Source: CAD feature listing. Evaluate the final solid. Frame: model axes, mm. Face numbers are marked on the shaded views. A direction names the side the tool comes from. Coordinates: 2 decimals unless noted, no trailing zeros. Write each loop counter-clockwise with the first axis right and the second up, starting at its lowest first coordinate (ties: lowest second). Pieces come first, ordered by that corner, then holes. Notation, with made-up numbers: (29.25, 71.5) - (43.25, 71.5) arc R19 ccw to (43.25, 93.5) - close; hole circle Ø3 at (6.5, 60.25). An arc over 180 degrees is marked (long way). One line per item, written item: value.
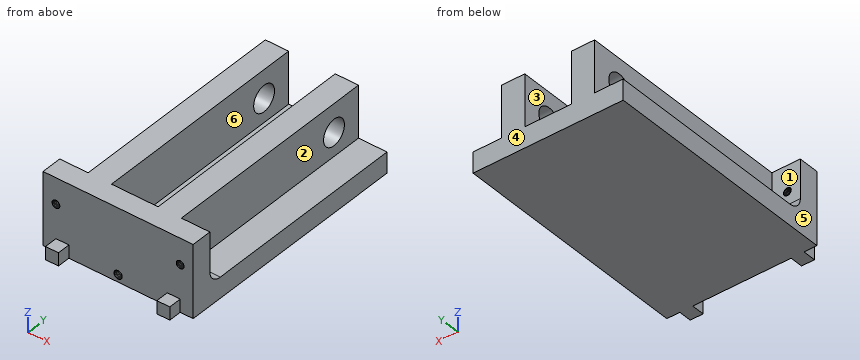
from build123d import *

# Parameters (mm, degrees)
SKETCH1_W           = 57.999998332
SKETCH1_H           = 28.000000864
BOSS_EXTRUDE1_DEPTH = 8
CUT_EXTRUDE2_REACH  = 43.097
CUT_EXTRUDE3_DEPTH  = 42.097445176
CUT_EXTRUDE4_DEPTH  = 42.097445176
SKETCH8_W           = 5.00000082
SKETCH8_H           = 4.999999888
BOSS_EXTRUDE2_DEPTH = 4.999995232
SKETCH9_W           = 5.00000082
SKETCH9_H           = 4.999999888
BOSS_EXTRUDE3_DEPTH = 4.999995232
BOSS_EXTRUDE4_DEPTH = 85
FILLET1_R           = 5
FILLET2_R           = 5
FILLET3_R           = 5
HOLE1_START         = -18
HOLE1_OUTLINE_R     = 5
HOLE1_DEPTH         = 36


# Read off the part's stored shape, not the designer's step: Hole1
with BuildPart() as part:
    # Sketch1 → Boss-Extrude1 (new body)
    with BuildSketch(Plane.XZ):
        with Locations((0, 14.000000432)):
            Rectangle(SKETCH1_W, SKETCH1_H)
    extrude(amount=BOSS_EXTRUDE1_DEPTH)

    # Sketch3 → Cut-Extrude2 (cut, up to next)
    with BuildSketch(Plane.XZ.offset(8), mode=Mode.PRIVATE) as cut_extrude2_sk1:
        Polygon((0, 4.350000061), (-0.277837098, 4.325692076), (-0.547232223, 4.253508057), (-0.79999998, 4.135640804), (-1.028459985, 3.975670785), (-1.225671032, 3.77845997), (-1.385641051, 3.550000023), (-1.503507956, 3.297232091), (-1.575691975, 3.027837025), (-1.59999996, 2.749999985), (-1.575691975, 2.472162945), (-1.503507956, 2.202768112), (-1.385641051, 1.949999947), (-1.225671032, 1.72154), (-1.028459985, 1.524328953), (-0.79999998, 1.36435905), (-0.547232223, 1.246492029), (-0.277837098, 1.17430801), (0, 1.150000026), (0.277837098, 1.17430801), (0.547232223, 1.246492029), (0.79999998, 1.36435905), (1.028459985, 1.524328953), (1.225671032, 1.72154), (1.385641051, 1.949999947), (1.503507956, 2.202768112), (1.575691975, 2.472162945), (1.59999996, 2.749999985), (1.575691975, 3.027837025), (1.503507956, 3.297232091), (1.385641051, 3.550000023), (1.225671032, 3.77845997), (1.028459985, 3.975670785), (0.79999998, 4.135640804), (0.547232223, 4.253508057), (0.277837098, 4.325692076), align=None)
    cut_extrude2_tool1 = extrude(cut_extrude2_sk1.sketch, amount=-CUT_EXTRUDE2_REACH, mode=Mode.PRIVATE) & part.part
    add(cut_extrude2_tool1.solids().sort_by_distance((0, -8, 2.75))[0], mode=Mode.SUBTRACT)

    # Sketch4 → Cut-Extrude3 (cut, through all)
    with BuildSketch(Plane.XZ.offset(8)):
        Polygon((-23.035820574, 16.850929707), (-22.850930691, 17.03581959), (-22.700959817, 17.249999568), (-22.590460256, 17.486970872), (-22.522790357, 17.739530653), (-22.500000894, 17.999999225), (-22.522790357, 18.26046966), (-22.590460256, 18.513029441), (-22.700959817, 18.750000745), (-22.850930691, 18.964180723), (-23.035820574, 19.149070606), (-23.250000551, 19.299039617), (-23.486969993, 19.409539178), (-23.739529774, 19.477209076), (-24.000000209, 19.500000402), (-24.260470644, 19.477209076), (-24.513030425, 19.409539178), (-24.749999866, 19.299039617), (-24.964179844, 19.149070606), (-25.149069726, 18.964180723), (-25.299040601, 18.750000745), (-25.409540161, 18.513029441), (-25.47721006, 18.26046966), (-25.499999523, 17.999999225), (-25.47721006, 17.739530653), (-25.409540161, 17.486970872), (-25.299040601, 17.249999568), (-25.149069726, 17.03581959), (-24.964179844, 16.850929707), (-24.749999866, 16.700960696), (-24.513030425, 16.590459272), (-24.260470644, 16.522789374), (-24.000000209, 16.499999911), (-23.739529774, 16.522789374), (-23.486969993, 16.590459272), (-23.250000551, 16.700960696), align=None)
    extrude(amount=-CUT_EXTRUDE3_DEPTH, mode=Mode.SUBTRACT)

    # Sketch5 → Cut-Extrude4 (cut, through all)
    with BuildSketch(Plane(origin=(0, -8, 0), x_dir=(-1, 0, 0), z_dir=(0, 1, 0))):
        Polygon((-23.486969993, 16.590459272), (-23.250000551, 16.700960696), (-23.035820574, 16.850929707), (-22.850930691, 17.03581959), (-22.700959817, 17.249999568), (-22.590460256, 17.486970872), (-22.522790357, 17.739530653), (-22.500000894, 17.999999225), (-22.522790357, 18.26046966), (-22.590460256, 18.513029441), (-22.700959817, 18.750000745), (-22.850930691, 18.964180723), (-23.035820574, 19.149070606), (-23.250000551, 19.299039617), (-23.486969993, 19.409539178), (-23.739529774, 19.477209076), (-24.000000209, 19.500000402), (-24.260470644, 19.477209076), (-24.513030425, 19.409539178), (-24.749999866, 19.299039617), (-24.964179844, 19.149070606), (-25.149069726, 18.964180723), (-25.299040601, 18.750000745), (-25.409540161, 18.513029441), (-25.47721006, 18.26046966), (-25.499999523, 17.999999225), (-25.47721006, 17.739530653), (-25.409540161, 17.486970872), (-25.299040601, 17.249999568), (-25.149069726, 17.03581959), (-24.964179844, 16.850929707), (-24.749999866, 16.700960696), (-24.513030425, 16.590459272), (-24.260470644, 16.522789374), (-24.000000209, 16.499999911), (-23.739529774, 16.522789374), align=None)
    extrude(amount=CUT_EXTRUDE4_DEPTH, mode=Mode.SUBTRACT)

    # Sketch8 → Boss-Extrude2 (add)
    with BuildSketch(Plane.XZ.offset(8)):
        with Locations((-21.499999799, 2.499999944)):
            Rectangle(SKETCH8_W, SKETCH8_H)
    extrude(amount=BOSS_EXTRUDE2_DEPTH)

    # Sketch9 → Boss-Extrude3 (add)
    with BuildSketch(Plane.XZ.offset(8)):
        with Locations((21.499999799, 2.499999944)):
            Rectangle(SKETCH9_W, SKETCH9_H)
    extrude(amount=BOSS_EXTRUDE3_DEPTH)

    # Sketch10 → Boss-Extrude4 (add)
    with BuildSketch(Plane(origin=(0, 0, 0), x_dir=(1, 0, 0), z_dir=(0, 1, 0))):
        Polygon((9, -8), (-9, -8), (-9, -28.000000864), (-18, -28.000000864), (-18, -8), (-28.999999166, -8), (-28.999999166, 0), (28.999999166, 0), (28.999999166, -8), (18, -8), (18, -28.000000864), (9, -28.000000864), align=None)
    extrude(amount=BOSS_EXTRUDE4_DEPTH)

    # Fillet1
    fillet1_edges = [part.edges().sort_by_distance(p)[0] for p in [
        (0, 0, 8),
    ]]
    fillet(fillet1_edges, radius=FILLET1_R)

    # Fillet2
    fillet2_edges = [part.edges().sort_by_distance(p)[0] for p in [
        (23.499999583, 0, 8),
    ]]
    fillet(fillet2_edges, radius=FILLET2_R)

    # Fillet3
    fillet3_edges = [part.edges().sort_by_distance(p)[0] for p in [
        (-23.499999583, 0, 8),
    ]]
    fillet(fillet3_edges, radius=FILLET3_R)

    # Hole1 outline → Hole1 (cut)
    with BuildSketch(Plane.YZ.offset(HOLE1_START)):
        with Locations((73.240950457, 17.082405748)):
            Circle(HOLE1_OUTLINE_R)
    extrude(amount=HOLE1_DEPTH, mode=Mode.SUBTRACT)


solid = part.part
1) Draft query along X for the marked faces 4, 5 and 6. Return one class per face: released by +X, released by -X, zero draft, split by the parting line, or undercut.
Values found:
face 4: zero draft
face 5: released by -X
face 6: undercut
2) Section query D-D on z = 6.75. Output: boundary loops of the cut face in (x, y).
Values found:
outline: (-29, -8) - (29, -8) - (29, 85) - (-29, 85) - close
3) Reachability of the marked faces 1, 2 and 3 from +Z, -Z, +X, -X, +Y, -Y: full face, straight path, thin tool, end or side. Return the list, or none.
Values found:
face 1: +Z, -X, +Y
face 2: +Z, +X, +Y
face 3: +Z, +Y
4) Material intervals for line 1 (X direction, y = 9.5, z = 15.75); line 2 (Y direction, x = 10, z = 17.5); line 3 (Z direction, x = -26, y = 73), sorted ascending.
Values found:
line 1: -18 to -9, 9 to 18
line 2: -8 to 68.26, 78.22 to 85
line 3: 0 to 8
5) Section query B-B on y = 55. Output: boundary loops of the cut face in (x, z), then the cut area to 3 significant figures.
Values found:
outline: (-29, 0) - (29, 0) - (29, 8) - (18, 8) - (18, 28) - (9, 28) - (9, 8) - (-9, 8) - (-9, 28) - (-18, 28) - (-18, 8) - (-29, 8) - close
area: 824 mm2
6) Section query A-A on z = 14. Output: boundary loops of the cut face in (x, y).
Values found:
outline: (-29, -8) - (29, -8) - (29, 0) - (18, 0) - (18, 69.3) - (9, 69.3) - (9, 0) - (-9, 0) - (-9, 69.3) - (-18, 69.3) - (-18, 0) - (-29, 0) - close; (-18, 77.18) - (-9, 77.18) - (-9, 85) - (-18, 85) - close; (9, 77.18) - (18, 77.18) - (18, 85) - (9, 85) - close
7) Section query C-C on x = -6.5. Output: boundary loops of the cut face in (y, z).
Values found:
outline: (-8, 0) - (85, 0) - (85, 8) - (5, 8) arc R5 cw to (0, 13) - (0, 28) - (-8, 28) - close
8) Contact query for flat-ended pins moving along their axis: P1, Ø16.5, axis at x = -0.5, z = 18, coming from the +Y side; P2, Ø5.5, axis at x = 25, z = 19.5, coming from the +Y side; P3, Ø1.5, axis at x = 20.5, y = -9.5, coming from the +Z side. Output: stop coordinate, or through.
Values found:
P1: y = 1.2
P2: y = 0
P3: z = 5
